Geometry check sheet. Reference: the model listing, model coordinates, mm. Coordinates: 2 decimals unless noted, no trailing zeros. Order: outer loops, then holes, each group sorted by start corner. A loop starts at its lowest first (then second) coordinate and runs counter-clockwise, first axis right, second up. Notation, with made-up numbers: (53.5, 42.25) - (86.5, 42.25) arc R32 cw to (86.5, 75.25) - close; hole circle Ø1 at (-0.5, 7). An arc over 180 degrees is marked (long way). Return JSON: item names as keys, results as strings. Group by question number.
Item 1: Scan lines: probe 1 along Y at (x, z) = (12.7, -24.6); probe 2 along Z at (x, y) = (3, 62); probe 3 along X at (y, z) = (397, -2). Record each from-to range of solid material in increasing order.
Item 2: Section check A-A on y = 203. Enter the section's corners in (x, z), then the cut area to 3 significant figures.
Item 3: Gauge pin test, flat end, axial feed: pin 1 (12 mm diameter, centred on x = 10, z = -9, fed in from +Y). Record the tip position at first contact, or that the pin passes through.
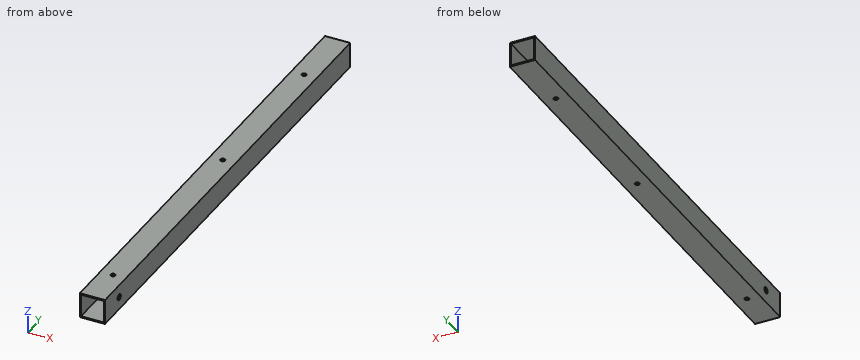
from build123d import *

# Parameters (mm, degrees)
SKETCH1_W           = 25.4
SKETCH1_H           = 25.4
BOSS_EXTRUDE1_DEPTH = 482.6
SKETCH2_R           = 2.286
CUT_EXTRUDE1_DEPTH  = 484.934995635
SKETCH3_R           = 2.286
CUT_EXTRUDE2_DEPTH  = 484.934995635
SKETCH4_R           = 2.286
CUT_EXTRUDE3_DEPTH  = 484.934995635
SKETCH9_R           = 3.175
CUT_EXTRUDE8_DEPTH  = 484.934995635


with BuildPart() as part:
    # Sketch1 → Boss-Extrude1 (new body)
    with BuildSketch(Plane(origin=(0, 0, 0), x_dir=(1, 0, 0), z_dir=(0, 1, 0))):
        with Locations((12.7, 12.7)):
            Rectangle(SKETCH1_W, SKETCH1_H)
        Polygon((1.27, 12.361459156), (1.27, 24.13), (12.7, 24.13), (24.13, 24.13), (24.13, 12.7), (24.13, 1.27), (12.7, 1.27), (1.27, 1.27), align=None, mode=Mode.SUBTRACT)
    extrude(amount=BOSS_EXTRUDE1_DEPTH)

    # Sketch2 → Cut-Extrude1 (cut, through all)
    with BuildSketch(Plane(origin=(0, 0, -25.4), x_dir=(-1, 0, 0), z_dir=(0, 0, -1))):
        with Locations((-12.7, 416.56)):
            Circle(SKETCH2_R)
    extrude(amount=-CUT_EXTRUDE1_DEPTH, mode=Mode.SUBTRACT)

    # Sketch3 → Cut-Extrude2 (cut, through all)
    with BuildSketch(Plane(origin=(0, 0, -25.4), x_dir=(-1, 0, 0), z_dir=(0, 0, -1))):
        with Locations((-12.7, 40.64)):
            Circle(SKETCH3_R)
    extrude(amount=-CUT_EXTRUDE2_DEPTH, mode=Mode.SUBTRACT)

    # Sketch4 → Cut-Extrude3 (cut, through all)
    with BuildSketch(Plane(origin=(0, 0, -25.4), x_dir=(-1, 0, 0), z_dir=(0, 0, -1))):
        with Locations((-12.7, 256.54)):
            Circle(SKETCH4_R)
    extrude(amount=-CUT_EXTRUDE3_DEPTH, mode=Mode.SUBTRACT)

    # Sketch9 → Cut-Extrude8 (cut, through all)
    with BuildSketch(Plane.ZY):
        with Locations((-12.7, 27.94)):
            Circle(SKETCH9_R)
    extrude(amount=-CUT_EXTRUDE8_DEPTH, mode=Mode.SUBTRACT)


solid = part.part
Computed:
{
 "1": {"probe 1": "y = 0 to 38.35, 42.93 to 254.25, 258.83 to 414.27, 418.85 to 482.6", "probe 2": "z = -25.4 to -24.13, -1.27 to 0", "probe 3": "x = 0 to 1.27, 24.13 to 25.4"},
 "2": {"outline": "(0, -25.4) - (25.4, -25.4) - (25.4, 0) - (0, 0) - close; hole (1.27, -24.13) - (24.13, -24.13) - (24.13, -1.27) - (1.27, -1.27) - close", "area": "123 mm²"},
 "3": {"pin 1": "passes through"}
}
